Can you work these out from the model? Positions are in its coordinate system, mm. A direction names the side the tool comes from. Give positions to 0.01 mm unless a question says otherwise; leave off trailing zeros. Loops run counter-clockwise (first coordinate to the right, second up) from the corner with the lowest first, then second, coordinate; pieces in that order, holes last.
Autodesk Fusion 360 part; units mm, degrees
sketch "Sketch1" plane through (0, 0, 0) normal (0, 0, 1) x (1, 0, 0)
  circle A0 centre (-190.0028, 38.6598) radius 2.5
  circle A1 centre (-223.4863, -19.3348) radius 2.5
  circle A2 centre (-156.5107, -19.3321) radius 2.5
  line L0 (-270.2459, -44.3327) -> (-191.7303, 91.6603)
  line L1 (-188.2662, 91.6603) -> (-109.7506, -44.3327)
  line L2 (-111.4826, -47.3327) -> (-268.5139, -47.3327)
  line L3 (-274.0245, -46.8774) -> (-272.6069, -49.3327)
  line L4 (-274.0245, -46.8774) -> (-191.4162, 96.2043)
  line L5 (-188.5801, 96.204) -> (-191.4221, 96.204)
  line L6 (-107.3967, -49.3327) -> (-105.9755, -46.8713)
  line L7 (-107.3967, -49.3327) -> (-272.6069, -49.3327)
  line L8 (-188.5801, 96.204) -> (-105.9755, -46.8713)
  arc A3 (-270.2459, -44.3327) -> (-268.5139, -47.3327) centre (-268.5139, -45.3327) ccw
  arc A4 (-188.2662, 91.6603) -> (-191.7303, 91.6603) centre (-189.9983, 90.6603) ccw
  arc A5 (-111.4826, -47.3327) -> (-109.7506, -44.3327) centre (-111.4826, -45.3327) ccw
  arc A6 (-219.1504, -3.8327) -> (-207.8921, -23.3327) centre (-207.8921, -10.3327) ccw
  arc A7 (-178.7399, 27.1603) -> (-201.2566, 27.1603) centre (-189.9983, 20.6603) ccw
  arc A8 (-172.1044, -23.3327) -> (-160.8461, -3.8327) centre (-172.1044, -10.3327) ccw
  arc A9 (-185.6681, 9.1603) -> (-194.3284, 9.1603) centre (-189.9983, 6.6603) ccw
  arc A10 (-200.0979, -0.8327) -> (-195.7678, -8.3327) centre (-195.7678, -3.3327) ccw
  arc A11 (-184.2287, -8.3327) -> (-179.8986, -0.8327) centre (-184.2287, -3.3327) ccw
  line L9 (-182.9361, 8.4283) -> (-173.4098, 13.9283)
  line L10 (-179.1666, 1.8993) -> (-169.6403, 7.3993)
  line L11 (-206.4769, 14.1788) -> (-197.0336, 8.5351)
  line L12 (-200.7511, 1.9755) -> (-210.1943, 7.6193)
  line L13 (-186.2287, -10.3327) -> (-186.2287, -21.3327)
  line L14 (-193.7678, -10.3327) -> (-193.7678, -21.3327)
  line L15 (-194.3284, 9.1603) -> (-194.2756, 9.2518)
  line L16 (-200.0451, -0.7412) -> (-200.0979, -0.8327)
  line L17 (-207.8921, -23.3327) -> (-195.7678, -23.3327)
  line L18 (-184.2287, -23.3327) -> (-172.1044, -23.3327)
  line L19 (-201.2566, 27.1603) -> (-207.1829, 16.8956)
  line L20 (-212.9524, 6.9025) -> (-219.1504, -3.8327)
  line L21 (-160.8461, -3.8327) -> (-166.9082, 6.6673)
  line L22 (-172.6777, 16.6603) -> (-178.7399, 27.1603)
  arc A12 (-185.6681, 9.1603) -> (-182.9361, 8.4283) centre (-183.9361, 10.1603) ccw
  arc A13 (-173.4098, 13.9283) -> (-172.6777, 16.6603) centre (-174.4098, 15.6603) ccw
  arc A14 (-166.9082, 6.6673) -> (-169.6403, 7.3993) centre (-168.6403, 5.6673) ccw
  arc A15 (-179.1666, 1.8993) -> (-179.8986, -0.8327) centre (-178.1666, 0.1673) ccw
  arc A16 (-184.2287, -8.3327) -> (-186.2287, -10.3327) centre (-184.2287, -10.3327) ccw
  arc A17 (-193.7678, -10.3327) -> (-195.7678, -8.3327) centre (-195.7678, -10.3327) ccw
  arc A18 (-200.0451, -0.7412) -> (-200.7511, 1.9755) centre (-201.7771, 0.2588) ccw
  arc A19 (-197.0336, 8.5351) -> (-194.2756, 9.2518) centre (-196.0076, 10.2518) ccw
  arc A20 (-207.1829, 16.8956) -> (-206.4769, 14.1788) centre (-205.4509, 15.8956) ccw
  arc A21 (-210.1943, 7.6193) -> (-212.9524, 6.9025) centre (-211.2204, 5.9025) ccw
  arc A22 (-195.7678, -23.3327) -> (-193.7678, -21.3327) centre (-195.7678, -21.3327) ccw
  arc A23 (-186.2287, -21.3327) -> (-184.2287, -23.3327) centre (-184.2287, -21.3327) ccw
  dimension "d1" = 5
  dimension "d2" = 5
  dimension "d3" = 5
  dimension "d5" = 120
  dimension "d11" = 2.842
  dimension "d12" = 120
  dimension "d13" = 60
  dimension "d16" = 120
  dimension "d17" = 120
  dimension "d18" = 120
  dimension "d19" = 2
  dimension "d20" = 2
  dimension "d21" = 2
  dimension "d22" = 2
  dimension "d23" = 60
  dimension "d24" = 60
  dimension "d25" = 24
  dimension "d26" = 24
  dimension "d27" = 24
  dimension "d28" = 13
  dimension "d32" = 5
  dimension "d34" = 2
  dimension "d35" = 2
  dimension "d36" = 2
  dimension "d37" = 2
  dimension "d38" = 2
  dimension "d39" = 2
  dimension "d40" = 2
  dimension "d41" = 2
extrude "Extrude1" add sketch "Sketch1" along normal blind 1.6 contours L0 L1 L2 A3 A4 A5
(1) Will these pins go through, and if not, where does the flat tip stop? P1, Ø4.5, axis at x = -156.51, y = -19.33, coming from the +Z side; P2, Ø0.5, axis at x = -199, z = 0.5, coming from the +Y side.
Returned:
P1: passes through
P2: stops at y = 79.5
(2) Suppose I cut it at D-D on z = 0.25. Give the number of separate pieces and of enclosed holes in the cut face, plus the area to 3 significant figures.
Returned:
separate pieces: 1
enclosed holes: 6
area: 9,750 mm2
(3) Suppose I cut it at A-A on y = 19.5. List the corners of the cut face in (x, z) for me.
Returned:
outline: (-233.39, 0) - (-205.68, 0) - (-205.68, 1.6) - (-233.39, 1.6) - close; (-174.32, 0) - (-146.6, 0) - (-146.6, 1.6) - (-174.32, 1.6) - close
(4) Suppose I cut it at C-C on x = -250.5. List the corners of the cut face in (y, z) for me, plus the area to 3 significant figures.
Returned:
outline: (-47.33, 0) - (-10.13, 0) - (-10.13, 1.6) - (-47.33, 1.6) - close
area: 59.5 mm2
(5) Thinking about a two-plate mould opening in X: for faces 1 (the flat face through (-191, 8, 0)), 2 (the flat face through (-149.56, 24.62, 0.79)), 3 (the cylindrical face through (-180, -6, 1)), which applies, pulls with the +X half, pulls with the -X half, needs draft (parallel to the pull), parting line crosses it, or undercut?
Returned:
face 1: needs draft
face 2: pulls with the +X half
face 3: undercut
(6) Suppose I cut it at B-B on y = 4. List the corners of the cut face in (x, z) for me, plus the area to 3 significant figures.
Returned:
outline: (-242.34, 0) - (-214.63, 0) - (-214.63, 1.6) - (-242.34, 1.6) - close; (-204.14, 0) - (-175.53, 0) - (-175.53, 1.6) - (-204.14, 1.6) - close; (-165.37, 0) - (-137.66, 0) - (-137.66, 1.6) - (-165.37, 1.6) - close
area: 134 mm2
(7) Please list where these lines run through material, in increasing order: probe 1 along X at (y, z) = (-5.5, 1.3); probe 2 along X at (y, z) = (-16, 1.5); probe 3 along X at (y, z) = (25.5, 1.25).
Returned:
probe 1: x = -247.83 to -219.96, -200.27 to -179.72, -160.04 to -132.17
probe 2: x = -253.89 to -219.59, -193.77 to -186.23, -160.4 to -126.11
probe 3: x = -229.93 to -202.22, -177.78 to -150.07
(8) Which directions (+Z, -Z, +X, -X, +Y, -Y) give clear straight access to the entire face, cutting with the end or side of a thin tool? Please do faces 4 (the flat face through (-205.41, 4.76, 0.79)), 5 (the flat face through (-191, 8, 1.6)).
Returned:
face 4: +Z, -Z
face 5: +Z, +X, -X, +Y, -Y
